Model file for the job. Use its own axes, mm. Give positions to 0.01 mm unless a question says otherwise; leave off trailing zeros. Write each loop counter-clockwise with the first axis right and the second up, starting at its lowest first coordinate (ties: lowest second). Pieces come first, ordered by that corner, then holes. Notation, with made-up numbers: (55, 18) - (101, 18) arc R23 ccw to (101, 42) - close; hole circle Ø11 at (-33.75, 73). An arc over 180 degrees is marked (long way). Use CSV: the item, a comma, the result in double quotes.
from build123d import *

# Parameters (mm, degrees)
F1_DEPTH = 311.15
F2_W     = 311.15
F2_H     = 19.05
F3_DEPTH = 311.151


with BuildPart() as f1:
    # F0 (on Front) → F1 (new body)
    with BuildSketch(Plane.XZ):
        Polygon((-311.15, 0), (0, 0), (0, 19.05), (-155.575, 34.925), (-311.15, 19.05), align=None)
    extrude(amount=-F1_DEPTH)

    # F2 (on face) → F3 (intersect, through all)
    with BuildSketch(Plane(origin=(-311.15, 0, 0), x_dir=(0, -1, 0), z_dir=(-1, 0, 0))):
        Polygon((-311.15, 19.05), (0, 19.05), (-155.575, 34.925), align=None)
        with Locations((-155.575, 9.525)):
            Rectangle(F2_W, F2_H)
    extrude(amount=-F3_DEPTH, mode=Mode.INTERSECT)


solid = f1.part
(1) Wall check: probe 1 along Z at (x, y) = (-69.5, 198); probe 2 along Z at (x, y) = (-245, 92.5). Give the ranges that are in metal, low to high. Write a range as [from, to].
Checked values:
probe 1,"z = [0, 26.14]"
probe 2,"z = [0, 25.8]"
(2) Saw through at A-A, the plane x = -91.5. List the corners of the cut face in (y, z).
Checked values:
outline,"(0, 0) - (311.15, 0) - (311.15, 19.05) - (219.65, 28.39) - (91.5, 28.39) - (0, 19.05) - close"
(3) Flat gauge pins, fed straight in: P1, Ø1, axis at x = -268, y = 63, coming from the +Z side; P2, Ø6, axis at x = -136.5, y = 71, coming from the +Z side; P3, Ø10, axis at x = -40, y = 125, coming from the +Z side. Where does each tip first touch, or does it go through?
Checked values:
P1,"stops at z = 23.5"
P2,"stops at z = 26.6"
P3,"stops at z = 23.64"
(4) Saw through at B-B, the plane z = 28. List the corners of the cut face in (x, y).
Checked values:
outline,"(-223.44, 87.71) - (-87.71, 87.71) - (-87.71, 223.44) - (-223.44, 223.44) - close"
(5) Saw through at C-C, the plane y = 273. List the corners of the cut face in (x, z).
Checked values:
outline,"(-311.15, 0) - (0, 0) - (0, 19.05) - (-38.15, 22.94) - (-273, 22.94) - (-311.15, 19.05) - close"
